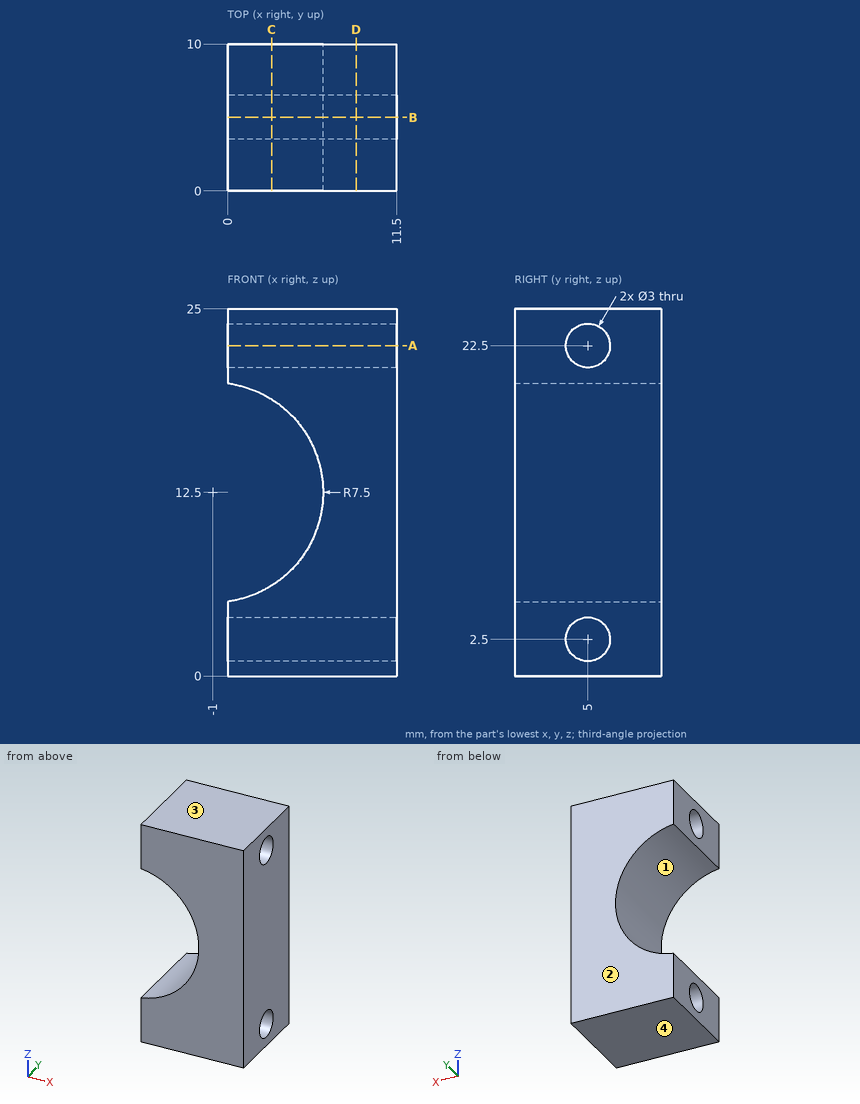
The drawing under review shows one solid part. Ordinate dimensions are in mm from its lowest x, y, z. Round coordinates to 2 decimals unless told otherwise and drop trailing zeros. Write each loop counter-clockwise with the first axis right and the second up, starting at its lowest first coordinate (ties: lowest second). Pieces come first, ordered by that corner, then holes.
(1) Mouldability with a two-part tool opening along Z and no side actions: class the marked faces 1, 2, 3 and 4 as +Z half, -Z half, draft (parallel to the pull), parting line (faces both ways), or undercut.
(2) Insertion check: pin 1 (1 mm diameter, centred on x = 3, z = 6, fed in from -Y); pin 2 (3 mm diameter, centred on y = 4.5, z = 10, fed in from -X). Each pin has a flat end and moves straight along its axis. Give the tip position at first contact, or say it passes through.
(3) We need section D-D on x = 8.75. Give the boundary of the cut face in (y, z), and give its area (3 significant figures).
(4) We need section C-C on x = 3. Give the boundary of the cut face in (y, z).
(5) We need section A-A on z = 22.5. Give the boundary of the cut face in (x, y).
(6) We need section B-B on y = 5. Give the boundary of the cut face in (x, z).
(7) Wall thickness on L1, parallel to Y at x = 5.5, z = 22.5; L2, parallel to Z at x = 0.5, y = 8.25; L3, parallel to X at y = 0.5, z = 8: over which ranges is each line inside the solid? List them lowest first.
Findings below:
1. face 1: undercut
1. face 2: draft
1. face 3: +Z half
1. face 4: -Z half
2. pin 1: stops at y = 0
2. pin 2: stops at x = 5.34
3. outline: (0, 0) - (10, 0) - (10, 25) - (0, 25) - close; hole circle Ø3 at (5, 2.5); hole circle Ø3 at (5, 22.5)
3. area: 236 mm2
4. outline: (0, 0) - (10, 0) - (10, 6.16) - (0, 6.16) - close; (0, 18.84) - (10, 18.84) - (10, 25) - (0, 25) - close; hole circle Ø3 at (5, 2.5); hole circle Ø3 at (5, 22.5)
5. outline: (0, 0) - (11.5, 0) - (11.5, 3.5) - (0, 3.5) - close; (0, 6.5) - (11.5, 6.5) - (11.5, 10) - (0, 10) - close
6. outline: (0, 0) - (11.5, 0) - (11.5, 1) - (0, 1) - close; (0, 4) - (11.5, 4) - (11.5, 21) - (0, 21) - (0, 19.93) arc R7.5 cw to (0, 5.07) - close; (0, 24) - (11.5, 24) - (11.5, 25) - (0, 25) - close
7. L1: y = 0 to 3.5, 6.5 to 10
7. L2: z = 0 to 5.15, 19.85 to 25
7. L3: x = 5 to 11.5
